Source: CAD feature listing. Evaluate the final solid. Frame: model axes, mm. A direction names the side the tool comes from. Round coordinates to 2 decimals unless told otherwise and drop trailing zeros. Order: outer loops, then holes, each group sorted by start corner. A loop starts at its lowest first (then second) coordinate and runs counter-clockwise, first axis right, second up. Notation, with made-up numbers: (15, -33) -> (58, -33) arc R18 ccw to (58, -25) -> close; hole circle Ø10 at (72, 76.25). An arc over 180 degrees is marked (long way). One line per item, written item: value. Start each with the question number.
1) Section B-B (x = 44). Return the cut outline in (y, z).
2) Reachability of faces 1 (the face through (67, 9, 10)), 2 (the face through (133.37, 2.406, 4.93)), 3 (the face through (2, 219, 10)), 4 (the face through (0, 137, 16)), 5 (the face through (135.651, 135, 14)) from +Z, -Z, +X, -X, +Y, -Y: full face, straight path, thin tool, end or side. Return the list, or none.
3) Section A-A (z = 5). Return the cut outline in (x, y), and give its area (4 significant figures).
4) Ray query, L1, parallel to Y at x = 108, z = 6; L2, parallel to X at y = 145, z = 30; L3, parallel to Z at x = 36, y = 176. Return the intervals inside material, ascending.
5) Mould query, pull axis X, two halves, no side actions, for faces 6 (the face through (133.246, 218.568, 4.93)), 7 (the face through (7.28, 213.44, 4.93)), 8 (the face through (67.29, 107.27, 36.56)), 9 (the face through (2.28, 218.44, 4.93)). Classes: pulls with the +X half, pulls with the -X half, needs draft (parallel to the pull), parting line crosses it, or undercut.
6) Pin query (flat end, axial travel): P1, Ø0.5, axis at x = 5.5, y = 211.5, coming from the +Z side; P2, Ø10, axis at x = 116.5, y = 39, coming from the -Z side; P3, Ø1.5, axis at x = 75.5, y = 214, coming from the -Z side. Return the tip coordinate at first contact, or that it passes through.
7) Section C-C (y = 186). Return the cut outline in (x, z), and give its area (3 significant figures).
Autodesk Inventor part; units mm, degrees
ref_plane "YZ Plane" through (0, 0, 0) normal (1, 0, 0) x (0, 1, 0)
ref_plane "XZ Plane" through (0, 0, 0) normal (0, 1, 0) x (-1, 0, 0)
ref_plane "XY Plane" through (0, 0, 0) normal (0, 0, 1) x (1, 0, 0)
sketch "Эскиз1" plane through (0, 0, 0) normal (0, 0, 1) x (1, 0, 0)
  line L0 (5, 13) -> (5, 207.8488)
  arc A0 (13, 215.8488) -> (5, 207.8488) centre (13, 207.8488) ccw
  line L1 (13, 215.8488) -> (122.6512, 215.8488)
  arc A1 (130.6512, 207.8488) -> (122.6512, 215.8488) centre (122.6512, 207.8488) ccw
  line L2 (130.6512, 207.8488) -> (130.6512, 13)
  arc A2 (122.6512, 5) -> (130.6512, 13) centre (122.6512, 13) ccw
  line L3 (13, 5) -> (122.6512, 5)
  arc A3 (5, 13) -> (13, 5) centre (13, 13) ccw
  arc A4 (127.6512, 0) -> (135.6512, 8) centre (127.6512, 8) ccw
  line L4 (135.6512, 8) -> (135.6512, 212.8488)
  arc A5 (135.6512, 212.8488) -> (127.6512, 220.8488) centre (127.6512, 212.8488) ccw
  line L5 (127.6512, 220.8488) -> (8, 220.8488)
  arc A6 (8, 220.8488) -> (0, 212.8488) centre (8, 212.8488) ccw
  line L6 (0, 8) -> (0, 212.8488)
  arc A7 (0, 8) -> (8, 0) centre (8, 8) ccw
  line L7 (127.6512, 0) -> (8, 0)
  point P0 (0, 0)
extrude "Выдавливание1" add sketch "Эскиз1" along normal blind 10
sketch "Эскиз2" plane through (0, 8, 0) normal (-1, 0, 0) x (0, 0, 1)
  line L0 (0, 212.8488) -> (10, 212.8488)
  line L1 (10, 212.8488) -> (40, 212.8488)
  arc A0 (10, -8) -> (40, 212.8488) centre (-486.9233, 171.9638) ccw
  line L2 (10, 212.8488) -> (10, -8)
  line L3 (10, 5) -> (10, -3)
  arc A1 (10, 5) -> (32.8436, 212.8488) centre (-556.7291, 172.466) ccw
  line L4 (0, 204.8488) -> (10, 204.8488)
  line L5 (10, 204.8488) -> (33.3371, 204.8488)
  point P0 (0, -8)
  dimension "d2" = 30
extrude "Выдавливание2" add sketch "Эскиз2" against normal blind 136.5 contours L1 A1 L5 L2 | L1 A0 L2 A1
sketch "Эскиз3" plane through (135.6512, 8, 0) normal (1, 0, 0) x (0, 0, -1)
  line L0 (-10, 5) -> (-10, 204.8488)
  arc A0 (-33.3371, 204.8488) -> (-10, 5) centre (556.7291, 172.466) ccw
  line L1 (-33.3371, 204.8488) -> (-10, 204.8488)
  point P0 (0, -8)
extrude "Выдавливание3" add sketch "Эскиз3" against normal blind 5
sketch "Эскиз4" plane through (0, 8, 0) normal (-1, 0, 0) x (0, 0, 1)
  arc A0 (10, 5) -> (33.3371, 204.8488) centre (-556.7291, 172.466) ccw
  line L0 (10, 204.8488) -> (10, 5)
  line L1 (10, 204.8488) -> (33.3371, 204.8488)
  point P0 (0, -8)
extrude "Выдавливание4" add sketch "Эскиз4" against normal blind 5
properties part number "krish"
Findings:
1. outline: (0, 0) -> (5, 0) -> (5, 10) -> (13, 10) arc R590.95 cw to (212.85, 33.34) -> (212.85, 10) -> (215.85, 10) -> (215.85, 0) -> (220.85, 0) -> (220.85, 40) arc R528.51 ccw to (0, 10) -> close
2. face 1: -Z
2. face 2: -Z, +X, -Y
2. face 3: -Z, -X, +Y
2. face 4: +Z, -Z, -X, +Y, -Y
2. face 5: -Z, +X
3. outline: (0, 8) arc R8 ccw to (8, 0) -> (127.65, 0) arc R8 ccw to (135.65, 8) -> (135.65, 212.85) arc R8 ccw to (127.65, 220.85) -> (8, 220.85) arc R8 ccw to (0, 212.85) -> close; hole (5, 13) arc R8 ccw to (13, 5) -> (122.65, 5) arc R8 ccw to (130.65, 13) -> (130.65, 207.85) arc R8 ccw to (122.65, 215.85) -> (13, 215.85) arc R8 ccw to (5, 207.85) -> close
3. area: 3,465 mm2
4. L1: 0 to 5, 215.85 to 220.85
4. L2: 0 to 5, 130.65 to 135.65
4. L3: 34.21 to 41.57
5. face 6: pulls with the +X half
5. face 7: undercut
5. face 8: needs draft
5. face 9: pulls with the -X half
6. P1: z = 40.66
6. P2: z = 15.79
6. P3: z = 10
7. outline: (0, 0) -> (5, 0) -> (5, 34.2) -> (130.65, 34.2) -> (130.65, 0) -> (135.65, 0) -> (135.65, 34.2) -> (136.5, 34.2) -> (136.5, 41.55) -> (0, 41.55) -> close
7. area: 1,350 mm2
